Autodesk Inventor part; units mm, degrees
ref_plane "YZ Plane" through (0, 0, 0) normal (1, 0, 0) x (0, 1, 0)
ref_plane "XZ Plane" through (0, 0, 0) normal (0, 1, 0) x (-1, 0, 0)
ref_plane "XY Plane" through (0, 0, 0) normal (0, 0, 1) x (1, 0, 0)
sketch "Sketch1" plane through (0, 0, 0) normal (0, 0, 1) x (1, 0, 0)
  line L0 (0, 0) -> (400, 0)
  line L1 (400, 0) -> (400, 500)
  line L2 (400, 500) -> (0, 500)
  line L3 (0, 500) -> (0, 0)
  dimension "d0" = 400
  dimension "d1" = 500
extrude "Extrusion1" add sketch "Sketch1" along normal blind 18
fillet "Fillet1" radius 150 1 edges at (400, 0, 9)
properties part number "Example" material "LMDF"
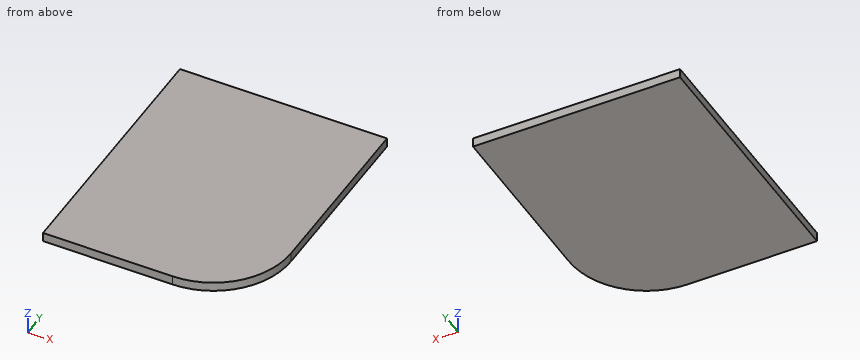
For this review, take the finished solid that the model builds, in its own axes (mm). Round coordinates to 2 decimals unless told otherwise and drop trailing zeros. Loops run counter-clockwise (first coordinate to the right, second up) from the corner with the lowest first, then second, coordinate; pieces in that order, holes last.
(1) We need section B-B (x = 329.5). Give the boundary of the cut face in (y, z).
Returned:
outline: (22.8, 0) - (500, 0) - (500, 18) - (22.8, 18) - close
(2) Clearance check with flat-ended pins moving along their axes: P1, Ø4, axis at x = 291.5, y = 196.5, coming from the -Z side; P2, Ø10, axis at y = 95.5, z = 5, coming from the +X side. State where each tip first meets the part, or that it passes through.
Returned:
P1: stops at z = 0
P2: stops at x = 391.6
(3) Wall thickness on line 1 along Y through (x, z) = (325, 10.75); line 2 along Y through (x, z) = (319, 7.75); line 3 along X through (y, z) = (133, 9): over which ranges is each line inside the solid? List them lowest first.
Returned:
line 1: y = 20.1 to 500
line 2: y = 16.81 to 500
line 3: x = 0 to 399.03
(4) We need section A-A (z = 13.75). Give the boundary of the cut face in (x, y).
Returned:
outline: (0, 0) - (250, 0) arc R150 ccw to (400, 150) - (400, 500) - (0, 500) - close
